Geometry check sheet. Reference: the model listing, model coordinates, mm. A direction names the side the tool comes from. Round coordinates to 2 decimals unless told otherwise and drop trailing zeros. Order: outer loops, then holes, each group sorted by start corner. A loop starts at its lowest first (then second) coordinate and runs counter-clockwise, first axis right, second up.
(1) Set-up check for faces 5 (the face through (-27, 2, 12)), 6 (the face through (0, -17.65, -14)), 7 (the face through (4, 0, -3.175)): record each of +Z, -Z, +X, -X, +Y, -Y from which the full face is reachable in a straight line by a thin tool's end or side.
(2) Sectioned sample at B-B (x = -16). Record the boundary of the cut face in (y, z) (3 decimals).
(3) Release check for a two-part mould opening along Y. For faces 1 (the face through (0, 27.81, 12)), 2 (the face through (0, 30.985, 6)), 3 (the face through (2.11, 2.55, -0.04)), 4 (the face through (-27, -21, -14)) record: +Y half, -Y half, draft (parallel to the pull), parting line (faces both ways), or undercut.
(4) Material ranges on line 1 along X through (y, z) = (-4, 18.5) (3 decimals); line 2 along Z through (x, y) = (16, -19.5) (3 decimals); line 3 along Y through (x, z) = (-6.75, 0.5) (3 decimals), recorded low to high.
(5) Go/stop test with flat-tipped pins: pin 1 (6 mm diameter, centred on x = 16, z = -13.175, fed in from +Y); pin 2 (7 mm diameter, centred on y = -22.5, z = -14.5, fed in from -X); pin 3 (3 mm diameter, centred on x = 5.5, y = 5.5, fed in from +Z) (3 decimals). Record where each tip stops, or that it passes through.
(6) Sectioned sample at A-A (y = 0). Record the boundary of the cut face in (x, z) (3 decimals).
(7) Sectioned sample at D-D (z = 9.5). Record the boundary of the cut face in (x, y) (3 decimals), plus the area to 3 significant figures.
(8) Sectioned sample at C-C (y = 7). Record the boundary of the cut face in (x, z) (3 decimals), plus the area to 3 significant figures.
from build123d import *

# Parameters (mm, degrees)
SKETCH1_W            = 48
SKETCH1_H            = 48
SKETCH1_R            = 1.75
SKETCH1_R_2          = 8.5
BOSS_EXTRUDE2_DEPTH  = 3.175
SKETCH2_W            = 14
SKETCH2_H            = 6.35
BOSS_EXTRUDE3_DEPTH  = 48
SKETCH3_W            = 48
SKETCH3_H            = 48
SKETCH3_R            = 17
BOSS_EXTRUDE4_DEPTH  = 5.499999938
M4_CLEARANCE_HOLE1_D = 4.5
SKETCH7_W            = 48
SKETCH7_H            = 6.35
BOSS_EXTRUDE5_DEPTH  = 2
BOSS_EXTRUDE6_DEPTH  = 3
SKETCH12_W           = 54
SKETCH12_H           = 48
CUT_EXTRUDE4_DEPTH   = 16
SKETCH15_W           = 3.175
SKETCH15_H           = 41.65
SKETCH15_H_2         = 3.175
SKETCH15_W_2         = 54
BOSS_EXTRUDE8_DEPTH  = 30
SKETCH16_W           = 54
SKETCH16_H           = 3.175
CUT_EXTRUDE5_DEPTH   = 45.565155952
SKETCH17_W           = 60.35
SKETCH17_H           = 30
BOSS_EXTRUDE9_DEPTH  = 10.16
SKETCH18_W           = 54
SKETCH18_H           = 10.16
CUT_EXTRUDE6_DEPTH   = 18.150000062


with BuildPart() as part:
    # Sketch1 → Boss-Extrude2 (new, symmetric)
    with BuildSketch(Plane.XY):
        Rectangle(SKETCH1_W, SKETCH1_H)
        with Locations((13.5, 0)):
            Circle(SKETCH1_R, mode=Mode.SUBTRACT)
        with Locations((-6.75, 11.691342951)):
            Circle(SKETCH1_R, mode=Mode.SUBTRACT)
        with Locations((-6.75, -11.691342951)):
            Circle(SKETCH1_R, mode=Mode.SUBTRACT)
        with Locations((-6, 0)):
            Circle(SKETCH1_R_2, mode=Mode.SUBTRACT)
    extrude(amount=BOSS_EXTRUDE2_DEPTH, both=True)

    # Sketch2 → Boss-Extrude3 (add)
    with BuildSketch(Plane(origin=(24, 0, 0), x_dir=(0, 0, -1), z_dir=(1, 0, 0))):
        with Locations((10.175, -20.825)):
            Rectangle(SKETCH2_W, SKETCH2_H)
    boss_extrude3 = extrude(amount=-BOSS_EXTRUDE3_DEPTH)

    # Sketch3 → Boss-Extrude4 (add)
    with BuildSketch(Plane.XY.offset(3.175)):
        Rectangle(SKETCH3_W, SKETCH3_H)
        Circle(SKETCH3_R, mode=Mode.SUBTRACT)
    boss_extrude4 = extrude(amount=BOSS_EXTRUDE4_DEPTH)

    # Mirror1: Boss-Extrude3, Boss-Extrude4 across plane
    add(boss_extrude3.mirror(Plane.XY))
    add(boss_extrude4.mirror(Plane.XY))

    # M4 Clearance Hole1 (through all)
    with Locations(Plane(origin=(0, -17.65, 0), x_dir=(1, 0, 0), z_dir=(0, 1, 0))):
        with Locations((-16, -13.175), (16, -13.175), (16, 13.175), (-16, 13.175)):
            Hole(M4_CLEARANCE_HOLE1_D / 2)

    # Sketch7 → Boss-Extrude5 (add)
    with BuildSketch(Plane.XY.offset(17.175)):
        with Locations((0, -20.825)):
            Rectangle(SKETCH7_W, SKETCH7_H)
    boss_extrude5 = extrude(amount=BOSS_EXTRUDE5_DEPTH)

    # Mirror2: Boss-Extrude5 across plane
    add(boss_extrude5.mirror(Plane.XY))

    # Sketch8 → Boss-Extrude6 (add)
    with BuildSketch(Plane.ZY.offset(24)):
        Polygon((-19.175, -17.65), (-19.175, -24), (19.175, -24), (19.175, -17.65), (8.674999938, -17.65), (8.674999938, 24), (-8.674999938, 24), (-8.674999938, -17.65), align=None)
    boss_extrude6 = extrude(amount=BOSS_EXTRUDE6_DEPTH)

    # Mirror3: Boss-Extrude6 across plane
    add(boss_extrude6.mirror(Plane(origin=(0, 0, 0), x_dir=(0, 0, 1), z_dir=(1, 0, 0))))

    # Sketch12 → Cut-Extrude4 (cut)
    with BuildSketch(Plane.XY.offset(19.175)):
        Rectangle(SKETCH12_W, SKETCH12_H)
    extrude(amount=-CUT_EXTRUDE4_DEPTH, mode=Mode.SUBTRACT)

    # Sketch15 → Boss-Extrude8 (add)
    with BuildSketch(Plane(origin=(0, 0, -8.674999938), x_dir=(-1, 0, 0), z_dir=(0, 0, -1))):
        Polygon((27, -24), (30.175, -24), (30.175, 17.65), (27, 17.65), (27, -17.65), align=None)
        with Locations((-28.5875, -3.175)):
            Rectangle(SKETCH15_W, SKETCH15_H)
        with Locations((-28.5875, 19.2375)):
            Rectangle(SKETCH15_W, SKETCH15_H_2)
        with Locations((0, 19.2375)):
            Rectangle(SKETCH15_W_2, SKETCH15_H_2)
        with Locations((28.5875, 19.2375)):
            Rectangle(SKETCH15_W, SKETCH15_H_2)
    extrude(amount=-BOSS_EXTRUDE8_DEPTH)

    # Sketch16 → Cut-Extrude5 (cut, through all)
    with BuildSketch(Plane.XY.offset(3.175)):
        with Locations((0, 22.4125)):
            Rectangle(SKETCH16_W, SKETCH16_H)
    extrude(amount=-CUT_EXTRUDE5_DEPTH, mode=Mode.SUBTRACT)

    # Sketch17 → Boss-Extrude9 (add)
    with BuildSketch(Plane(origin=(0, 20.825, 0), x_dir=(1, 0, 0), z_dir=(0, 1, 0))):
        with Locations((0, -6.325000062)):
            Rectangle(SKETCH17_W, SKETCH17_H)
    extrude(amount=BOSS_EXTRUDE9_DEPTH)

    # Sketch18 → Cut-Extrude6 (cut)
    with BuildSketch(Plane.XY.offset(21.325000062)):
        with Locations((0, 22.73)):
            Rectangle(SKETCH18_W, SKETCH18_H)
    extrude(amount=-CUT_EXTRUDE6_DEPTH, mode=Mode.SUBTRACT)


solid = part.part
Answer below:
1. face 5: +Z, -Y
1. face 6: -Z, +X, -X, +Y
1. face 7: -Z
2. outline: (-24, -19.175) - (-17.65, -19.175) - (-17.65, -15.425) - (-24, -15.425) - close; (-24, -10.925) - (-17.65, -10.925) - (-17.65, -8.675) - (-5.745, -8.675) - (-5.745, -3.175) - (5.745, -3.175) - (5.745, -8.675) - (30.985, -8.675) - (30.985, 21.325) - (27.81, 21.325) - (27.81, 3.175) - (-24, 3.175) - close
3. face 1: -Y half
3. face 2: +Y half
3. face 3: undercut
3. face 4: draft
4. line 1: x = -30.175 to -27, 27 to 30.175
4. line 2: z = -19.175 to -15.425, -10.925 to 3.175
4. line 3: y = -24 to -13.441, -9.941 to -8.467, 8.467 to 9.941, 13.441 to 30.985
5. pin 1: stops at y = -17.65
5. pin 2: stops at x = -27
5. pin 3: stops at z = 3.175
6. outline: (-30.175, -8.675) - (-17, -8.675) - (-17, -3.175) - (-14.5, -3.175) - (-14.5, 3.175) - (-27, 3.175) - (-27, 21.325) - (-30.175, 21.325) - close; (2.5, -3.175) - (11.75, -3.175) - (11.75, 3.175) - (2.5, 3.175) - close; (15.25, -3.175) - (17, -3.175) - (17, -8.675) - (30.175, -8.675) - (30.175, 21.325) - (27, 21.325) - (27, 3.175) - (15.25, 3.175) - close
7. outline: (-30.175, -24) - (-27, -24) - (-27, 27.81) - (27, 27.81) - (27, -24) - (30.175, -24) - (30.175, 30.985) - (-30.175, 30.985) - close
7. area: 521 mm2
8. outline: (-30.175, -8.675) - (-15.492, -8.675) - (-15.492, -3.175) - (-10.822, -3.175) - (-10.822, 3.175) - (-27, 3.175) - (-27, 21.325) - (-30.175, 21.325) - close; (-1.178, -3.175) - (15.492, -3.175) - (15.492, -8.675) - (30.175, -8.675) - (30.175, 21.325) - (27, 21.325) - (27, 3.175) - (-1.178, 3.175) - close
8. area: 599 mm2
